Source: CAD feature listing. Evaluate the final solid. Frame: model axes, mm. Give positions to 0.01 mm unless a question says otherwise; leave off trailing zeros. Write each loop counter-clockwise with the first axis right and the second up, starting at its lowest first coordinate (ties: lowest second). Pieces come first, ordered by that corner, then holes. Notation, with made-up numbers: M 1,63 L 55,63 A19 cw 55,80 Z; hole C 60,16 d2. An arc over 180 degrees is marked long. Return JSON: item names as keys, results as strings.
```python
from build123d import *

# Parameters (mm, degrees)
SKETCH1_R           = 2.1828125
BOSS_EXTRUDE1_DEPTH = 1.5875


with BuildPart() as part:
    # Sketch1 → Boss-Extrude1 (new body)
    with BuildSketch(Plane(origin=(0, 0, 0), x_dir=(1, 0, 0), z_dir=(0, 1, 0))):
        with BuildLine():
            Line((2.54, 0), (374.867897552, 0))
            ThreePointArc((374.867897552, 0), (377.214551564, -1.567984082), (376.663948776, -4.336051224))
            Line((376.663948776, -4.336051224), (330.943948776, -50.056051224))
            ThreePointArc((330.943948776, -50.056051224), (330.11991347, -50.606654013), (329.147897552, -50.8))
            Line((329.147897552, -50.8), (2.54, -50.8))
            ThreePointArc((2.54, -50.8), (0.743948776, -50.056051224), (0, -48.26))
            Line((0, -48.26), (0, -2.54))
            ThreePointArc((0, -2.54), (0.743948776, -0.743948776), (2.54, 0))
        make_face()
        with Locations((6.35, -6.35)):
            Circle(SKETCH1_R, mode=Mode.SUBTRACT)
        with Locations((19.05, -6.35)):
            Circle(SKETCH1_R, mode=Mode.SUBTRACT)
        with Locations((146.05, -6.35)):
            Circle(SKETCH1_R, mode=Mode.SUBTRACT)
        with Locations((158.75, -6.35)):
            Circle(SKETCH1_R, mode=Mode.SUBTRACT)
        with Locations((349.25, -6.35)):
            Circle(SKETCH1_R, mode=Mode.SUBTRACT)
        with Locations((361.95, -6.35)):
            Circle(SKETCH1_R, mode=Mode.SUBTRACT)
        with Locations((234.95, -6.35)):
            Circle(SKETCH1_R, mode=Mode.SUBTRACT)
    extrude(amount=BOSS_EXTRUDE1_DEPTH)


solid = part.part
```
1) Line query: line 1 (Z direction, x = 234.95, y = 1.3); line 2 (Z direction, x = 361.95, y = 0.4); line 3 (X direction, y = 0.9, z = 38.5). Output: solid intervals per line, ascending. Write a range as [from, to].
Numbers:
{"line 1": "z = [0, 4.17], [8.53, 50.8]", "line 2": "z = [0, 4.17], [8.53, 19.05]", "line 3": "x = [0, 342.5]"}
2) Cut plane B-B, the plane z = 23. Return the cut outline in (x, y), then the cut area to 3 significant figures.
Numbers:
{"outline": "M 0,0 L 358,0 L 358,1.59 L 0,1.59 Z", "area": "568 mm²"}
3) Cut plane A-A, the plane y = 0.9. Return the cut outline in (x, z), then the cut area to 3 significant figures.
Numbers:
{"outline": "M 0,2.54 A2.54 ccw 2.54,0 L 374.87,0 A2.54 ccw 376.66,4.34 L 330.94,50.06 A2.54 ccw 329.15,50.8 L 2.54,50.8 A2.54 ccw 0,48.26 Z; hole C 6.35,6.35 d4.37; hole C 19.05,6.35 d4.37; hole C 146.05,6.35 d4.37; hole C 158.75,6.35 d4.37; hole C 234.95,6.35 d4.37; hole C 349.25,6.35 d4.37; hole C 361.95,6.35 d4.37", "area": "17,900 mm²"}
